Read the model definition and answer for the solid it produces. Units are mm, in the model's axes. A direction names the side the tool comes from. Coordinates: 2 decimals unless noted, no trailing zeros. Loops run counter-clockwise (first coordinate to the right, second up) from the corner with the lowest first, then second, coordinate; pieces in that order, holes last.
Q1. Section C-C (z = -33.25) is taken. Give the vertices of the cut face in (x, y), then the cut area to 3 significant figures.
Q2. Section A-A (y = 5) is taken. Give the vertices of the cut face in (x, z).
Q3. The mould has two halves that part along X. Classify faces 4 (the face through (-0.041, 10, -25)), 5 (the face through (-73.92, 3, -31)), 6 (the face through (-7.29, 2.77, -15.82)): pulls with the +X half, pulls with the -X half, needs draft (parallel to the pull), parting line crosses it, or undercut.
Q4. Straight lines are drawn through the part: line 1 (Z direction, x = -51.5, y = 9.25); line 2 (X direction, y = 3.25, z = -33.5); line 3 (Y direction, x = -25.5, z = -34.5). For each, find the intervals that lie inside material, in ascending order.
Q5. Section D-D (x = -39) is taken. Give the vertices of the cut face in (y, z).
Q6. Section B-B (x = -17) is taken. Give the vertices of the cut face in (y, z), then the cut area to 3 significant figures.
Q7. Which of the six approach directions +Z, -Z, +X, -X, +Y, -Y give full straight-line access (tool end or side, diameter ignored) to faces 1 (the face through (0.795, 9, -25)), 2 (the face through (-7.72, 9.55, -33.13)), 3 (the face through (-30.641, 2.766, -16.685))?
Q8. Flat-ended cylindrical pins translate along their axes: P1, Ø7, axis at y = 11.5, z = -25.5, coming from the -X side; P2, Ø1.7, axis at y = 2.5, z = -18, coming from the +X side; P3, Ø6, axis at y = 9, z = -35, coming from the -X side. Find the tip coordinate at first contact, or state that the pin passes through.
from build123d import *

# Parameters (mm, degrees)
SKETCH2_W           = 23.364084101
SKETCH2_H           = 11.930596137
BOSS_EXTRUDE1_DEPTH = 2.54
SKETCH3_W           = 102.155729419
SKETCH3_H           = 1.194871536
BOSS_EXTRUDE3_DEPTH = 20.32
SCALE1_SCALE        = 0.6


with BuildPart() as part:
    # Sketch2 → Boss-Extrude1 (new body)
    with BuildSketch(Plane(origin=(0, 0, 0), x_dir=(1, 0, 0), z_dir=(0, 1, 0))):
        Polygon((0, 48.840877934), (27.34094948, 29.702213298), (27.34094948, 19.138664636), (0, 0), (-102.155729419, 0), (-102.155729419, 48.840877934), align=None)
        Polygon((-97.184647696, 5.095358767), (-97.184647696, 17.025954903), (-73.820563595, 17.025954903), align=None, mode=Mode.SUBTRACT)
        with Locations((-85.502605646, 35.667511367)):
            Rectangle(SKETCH2_W, SKETCH2_H, mode=Mode.SUBTRACT)
        Polygon((-65.369724665, 41.632809435), (-65.369724665, 29.702213298), (-37.780221099, 41.632809435), align=None, mode=Mode.SUBTRACT)
        Polygon((-12.676258395, 30.777041779), (-12.676258395, 41.632809435), (-37.780221099, 30.777041779), align=None, mode=Mode.SUBTRACT)
        Polygon((-65.369724665, 17.025954903), (-65.369724665, 5.095358767), (-88.236700593, 5.095358767), align=None, mode=Mode.SUBTRACT)
        Polygon((-56.670331649, 17.025954903), (-56.670331649, 5.095358767), (-37.780221099, 17.025954903), align=None, mode=Mode.SUBTRACT)
        Polygon((-37.780221099, 5.095358767), (-12.676258395, 5.095358767), (-12.676258395, 17.025954903), align=None, mode=Mode.SUBTRACT)
    extrude(amount=BOSS_EXTRUDE1_DEPTH)

    # Sketch3 → Boss-Extrude3 (add)
    with BuildSketch(Plane(origin=(0, 2.54, 0), x_dir=(1, 0, 0), z_dir=(0, 1, 0))):
        Polygon((-102.155729419, 48.840877934), (0, 48.840877934), (27.34094948, 29.702213298), (27.34094948, 19.138664636), (25.946282646, 19.138664636), (25.946282646, 29.702213298), (0, 47.646006398), (-102.155729419, 47.646006398), align=None)
        with Locations((-51.07786471, 0.597435768)):
            Rectangle(SKETCH3_W, SKETCH3_H)
    extrude(amount=BOSS_EXTRUDE3_DEPTH)


with BuildPart() as part_1:
    # Scale1: scaled about (-39.022733584, 5.036168927, -24.995733367)
    add(part.part.scale(SCALE1_SCALE).moved(Location((-15.609093434, 2.014467571, -9.998293347))))


solid = part_1.part
Numbers:
1. outline: (-76.9, 2.01) - (-73.92, 2.01) - (-73.92, 3.54) - (-76.9, 3.54) - close; (-59.9, 2.01) - (-54.83, 2.01) - (-54.83, 3.54) - (-59.9, 3.54) - close; (-42.27, 2.01) - (-27.21, 2.01) - (-27.21, 3.54) - (-42.27, 3.54) - close; (-23.21, 2.01) - (-6.96, 2.01) - (-6.96, 15.73) - (-7.89, 15.73) - (-7.89, 3.54) - (-23.21, 3.54) - close
1. area: 71.4 mm2
2. outline: (-76.9, -39.3) - (-15.61, -39.3) - (0.8, -27.82) - (0.8, -21.48) - (-0.04, -21.48) - (-0.04, -27.82) - (-15.61, -38.59) - (-76.9, -38.59) - close; (-76.9, -10.72) - (-15.61, -10.72) - (-15.61, -10) - (-76.9, -10) - close
3. face 4: pulls with the -X half
3. face 5: undercut
3. face 6: pulls with the +X half
4. line 1: z = -39.3 to -38.59, -10.72 to -10
4. line 2: x = -76.9 to -73.92, -59.9 to -54.83, -41.7 to -26.63, -23.21 to -7.32
4. line 3: y = 2.01 to 3.54
5. outline: (2.01, -39.3) - (15.73, -39.3) - (15.73, -38.59) - (3.54, -38.59) - (3.54, -34.98) - (2.01, -34.98) - close; (2.01, -34.67) - (3.54, -34.67) - (3.54, -20.21) - (2.01, -20.21) - close; (2.01, -19.76) - (3.54, -19.76) - (3.54, -10.72) - (15.73, -10.72) - (15.73, -10) - (2.01, -10) - close
6. outline: (2.01, -39.3) - (15.73, -39.3) - (15.73, -38.59) - (3.54, -38.59) - (3.54, -10.72) - (15.73, -10.72) - (15.73, -10) - (2.01, -10) - close
6. area: 62.1 mm2
7. face 1: +Z, -Z, +X, +Y, -Y
7. face 2: +Z, -X, +Y
7. face 3: +Y, -Y
8. P1: stops at x = -1.75
8. P2: stops at x = -2.96
8. P3: stops at x = -14.76
